The listing builds one solid part. Answer for the finished solid, in the listing's coordinates (mm). A direction names the side the tool comes from. Round coordinates to 2 decimals unless told otherwise and drop trailing zeros. Loops run counter-clockwise (first coordinate to the right, second up) from the corner with the lowest first, then second, coordinate; pieces in that order, holes last. Notation, with made-up numbers: (0.5, 37) -> (19.5, 37) arc R33 cw to (19.5, 69) -> close; hole circle Ø7 at (2.25, 82.25). An arc over 180 degrees is marked (long way). Use a Markdown table: item, result. Add a question column.
Q1. Which of the six approach directions +Z, -Z, +X, -X, +Y, -Y give full straight-line access (tool end or side, diameter ignored) to faces 5 (the flat face through (-5, 6.6, -4)), 6 (the flat face through (-4.5, 27, 4)), 7 (the cylindrical face through (-0.74, 9, 3.32))?
Q2. Section A-A on y = 36 is taken. Give the vertices of the cut face in (x, z).
Q3. Given pin 1 Ø1 at (x, y) = (-1.5, 31.5) entering from +Z; pin 2 Ø11 at (y, z) = (36, 0) entering from +X; pin 3 Ø10 at (y, z) = (16.5, 2.5) entering from +X; pin 4 Ø5 at (x, y) = (-2, 10) entering from -Z, each flat-ended and moving along its own axis, determine where each tip first touches the part or whether it passes through.
Q4. Section B-B on y = 3.5 is taken. Give the vertices of the cut face in (x, z) (3 decimals), then the cut area to 3 significant figures.
Q5. For a pull along Z with two mould halves and no side action, classify faces 1 (the flat face through (-5.193, 21.561, -0.061)), 2 (the flat face through (-4.25, 41, 6)), 3 (the cylindrical face through (0.1, 3, 7.9)), 4 (the cylindrical face through (-0.275, 15.016, -6.244)) as released by +Z, released by -Z, zero draft, split by the parting line, or undercut.
Q6. Section C-C on y = 14 is taken. Give the vertices of the cut face in (x, z).
Q7. Consider line 1 (Y direction, x = 3.75, z = -5.75); line 2 (X direction, y = 27, z = -4.25); line 3 (Y direction, x = 4.45, z = 0). Determine where each line is inside the solid, lowest interval first.
from build123d import *

# Parameters (mm, degrees)
SKETCH2_OUTSIDE_W        = 37.758
SKETCH2_OUTSIDE_H        = 37.758
CUT_EXTRUDE1_DEPTH       = 6.6
SKETCH3_OUTSIDE_W        = 37.758
SKETCH3_OUTSIDE_H        = 37.758
SKETCH3_OUTSIDE_W_2      = 9
SKETCH3_OUTSIDE_H_2      = 24
CUT_EXTRUDE2_DEPTH       = 31.630866785
SKETCH4_R                = 9.25
SKETCH4_R_2              = 7.25
CUT_EXTRUDE3_DEPTH       = 0.25
CUT_EXTRUDE4_START       = -0.25
SKETCH5_R                = 9.25
SKETCH5_R_2              = 7.25
CUT_EXTRUDE4_DEPTH       = 0.25
DOME2_FACE_RADIUS        = 7.25
DOME2_HEIGHT             = 3.8
FILLET1_R                = 1
FILLET2_R                = 0.25
CUT_EXTRUDE10_DEPTH      = 10.2995
M8_TAPPED_HOLE1_D        = 6.8
M8_TAPPED_HOLE1_DEPTH    = 22.25
M8_TAPPED_HOLE1_TIP      = 2.042926105
CUT_EXTRUDE11_DEPTH      = 51.168615687
CUT_EXTRUDE11_DEPTH_BACK = 51.168615687
SKETCH6_R                = 7.25


# Read off the part's stored shape, not the designer's step: Dome1
with BuildPart() as part:
    # Sketch1 → Revolve1 (revolve)
    with BuildSketch(Plane(origin=(0, 0, 0), x_dir=(0, 0, -1), z_dir=(1, 0, 0)), mode=Mode.PRIVATE) as revolve1_sk:
        with BuildLine():
            Line((0, 0), (7.9, 0))
            Line((7.9, 0), (7.9, 6.6))
            Line((7.9, 6.6), (6.25, 6.6))
            Line((6.25, 6.6), (6.25, 23.2))
            Line((6.25, 23.2), (10.245555029, 29.752712416))
            ThreePointArc((10.245555029, 29.752712416), (10.463447114, 41.875055276), (0, 48))
            Line((0, 48), (0, 0))
        make_face()
    revolve(revolve1_sk.sketch.rotate(Axis((0, 48, 0), (0, -1, 0)), 180), axis=Axis((0, 48, 0), (0, -1, 0)))

    # Sketch2 outside → Cut-Extrude1 (cut)
    with BuildSketch(Plane(origin=(0, 0, 0), x_dir=(-1, 0, 0), z_dir=(0, -1, 0))):
        Rectangle(SKETCH2_OUTSIDE_W, SKETCH2_OUTSIDE_H)
        with BuildLine():
            Line((-6.925, 3.801890977), (-6.925, -3.801890977))
            ThreePointArc((-6.925, -3.801890977), (0, -7.9), (6.925, -3.801890977))
            Line((6.925, -3.801890977), (6.925, 3.801890977))
            ThreePointArc((6.925, 3.801890977), (0, 7.9), (-6.925, 3.801890977))
        make_face(mode=Mode.SUBTRACT)
    extrude(amount=-CUT_EXTRUDE1_DEPTH, mode=Mode.SUBTRACT)

    # Sketch3 outside → Cut-Extrude2 (cut, through all)
    with BuildSketch(Plane(origin=(0, 22.5, 0), x_dir=(-1, 0, 0), z_dir=(0, -1, 0))):
        Rectangle(SKETCH3_OUTSIDE_W, SKETCH3_OUTSIDE_H)
        Rectangle(SKETCH3_OUTSIDE_W_2, SKETCH3_OUTSIDE_H_2, mode=Mode.SUBTRACT)
    extrude(amount=-CUT_EXTRUDE2_DEPTH, mode=Mode.SUBTRACT)

    # Sketch4 → Cut-Extrude3 (cut)
    with BuildSketch(Plane(origin=(4.5, 0, 0), x_dir=(0, 0, -1), z_dir=(1, 0, 0))):
        with Locations((0, 36)):
            Circle(SKETCH4_R)
        with Locations((0, 36)):
            Circle(SKETCH4_R_2, mode=Mode.SUBTRACT)
    extrude(amount=-CUT_EXTRUDE3_DEPTH, mode=Mode.SUBTRACT)

    # Sketch5 → Cut-Extrude4 (cut)
    with BuildSketch(Plane.ZY.offset(4.5).offset(CUT_EXTRUDE4_START)):
        with Locations(Location((0, 36, 0), (0, 0, 180))):
            Circle(SKETCH5_R)
        with Locations(Location((0, 36, 0), (0, 0, 180))):
            Circle(SKETCH5_R_2, mode=Mode.SUBTRACT)
    extrude(amount=CUT_EXTRUDE4_DEPTH, mode=Mode.SUBTRACT)

    # Dome1 outline → Dome1 (revolve)
    with BuildSketch(Plane(origin=(0, 36, 0), x_dir=(0, 1, 0), z_dir=(0, 0, -1))):
        with BuildLine():
            Line((0, -4.499999993), (0, -8.3))
            ThreePointArc((0, -8.3), (4.092752745, -7.292422991), (7.250000005, -4.499999993))
            Line((7.250000005, -4.499999993), (0, -4.499999993))
        make_face()
    revolve(axis=Axis((0, 36, 0), (1, 0, 0)))

    # Dome2: a dome of height H over a round flat face of radius A is a cap of a sphere of radius (A * A + H * H) / (2 * H)
    dome2_r = (DOME2_FACE_RADIUS * DOME2_FACE_RADIUS + DOME2_HEIGHT * DOME2_HEIGHT) / (2 * DOME2_HEIGHT)
    dome2_base = Plane((4.5, 36, 0), z_dir=(1, 0, 0))
    with Locations(dome2_base.offset(DOME2_HEIGHT - dome2_r)):
        dome2_ball = Sphere(dome2_r, mode=Mode.PRIVATE)
    add(split(dome2_ball, bisect_by=dome2_base, keep=Keep.TOP, mode=Mode.PRIVATE))

    # Fillet1
    # the kernel refuses this fillet: 1 mm, written as the material it takes off along each edge
    with BuildSketch(Plane(origin=(0, 6.6, 0), x_dir=(-0.9669082627273712, 0, 0.25512430591681584), z_dir=(0.25512430591681584, 0, 0.9669082627273712))) as fillet1_piece_1:
        with BuildLine():
            CenterArc((7.9 - FILLET1_R, FILLET1_R), FILLET1_R, 270, 90)
            Line((7.9, FILLET1_R), (7.9 + FILLET1_R * 0.02, FILLET1_R))
            Line((7.9 + FILLET1_R * 0.02, FILLET1_R), (7.9 + FILLET1_R * 0.02, -FILLET1_R * 0.02))
            Line((7.9 + FILLET1_R * 0.02, -FILLET1_R * 0.02), (7.9 - FILLET1_R, -FILLET1_R * 0.02))
            Line((7.9 - FILLET1_R, -FILLET1_R * 0.02), (7.9 - FILLET1_R, 0))
        make_face()
    revolve(axis=Axis((0, 6.6, 0), (0, -1, 0)), revolution_arc=209.561901965, mode=Mode.SUBTRACT)
    with BuildSketch(Plane(origin=(0, 6.6, 0), x_dir=(-0.9669082627273712, 0, -0.2551243059168157), z_dir=(0.2551243059168157, 0, -0.9669082627273712))) as fillet1_piece_2:
        with BuildLine():
            CenterArc((7.9 - FILLET1_R, -FILLET1_R), FILLET1_R, 360, 90)
            Line((7.9, -FILLET1_R), (7.9 + FILLET1_R * 0.02, -FILLET1_R))
            Line((7.9 + FILLET1_R * 0.02, -FILLET1_R), (7.9 + FILLET1_R * 0.02, FILLET1_R * 0.02))
            Line((7.9 + FILLET1_R * 0.02, FILLET1_R * 0.02), (7.9 - FILLET1_R, FILLET1_R * 0.02))
            Line((7.9 - FILLET1_R, FILLET1_R * 0.02), (7.9 - FILLET1_R, 0))
        make_face()
    revolve(axis=Axis((0, 6.6, 0), (0, 1, 0)), revolution_arc=209.561901965, mode=Mode.SUBTRACT)

    # Fillet2
    fillet2_edges = [part.edges().sort_by_distance(p)[0] for p in [
        (0, 0, -7.9),
        (0, 0, 7.9),
        (6.925, 0, 0),
        (-6.925, 0, 0),
    ]]
    fillet(fillet2_edges, radius=FILLET2_R)

    # Sketch11 → Cut-Extrude10 (cut, symmetric)
    with BuildSketch(Plane(origin=(0, 0, 0), x_dir=(-1, 0, 0), z_dir=(0, 0, -1))):
        Polygon((-6.25, 22.5), (-4.5, 22.5), (-6.25, 20.127174391), align=None)
        Polygon((4.5, 22.5), (6.25, 22.5), (6.25, 20.127174391), align=None)
    extrude(amount=CUT_EXTRUDE10_DEPTH, both=True, mode=Mode.SUBTRACT)

    # M8 Tapped Hole1
    with Locations(Plane(origin=(0, -4.5, 0), x_dir=(-1, 0, 0), z_dir=(0, -1, 0))):
        with Locations((0, 0)):
            Hole(M8_TAPPED_HOLE1_D / 2, depth=M8_TAPPED_HOLE1_DEPTH)
            with Locations((0, 0, -(M8_TAPPED_HOLE1_DEPTH + M8_TAPPED_HOLE1_TIP / 2))):  # 118° drill point
                Cone(0, M8_TAPPED_HOLE1_D / 2, M8_TAPPED_HOLE1_TIP, mode=Mode.SUBTRACT)

    # Sketch6 → Cut-Extrude11 (cut, two sides: drawn at the far end of the back side and taken through both)
    with BuildSketch(Plane(origin=(0, 0, 0), x_dir=(0, 0, -1), z_dir=(1, 0, 0)).offset(-CUT_EXTRUDE11_DEPTH_BACK)):
        with Locations((0, 36)):
            Circle(SKETCH6_R)
    extrude(amount=CUT_EXTRUDE11_DEPTH + CUT_EXTRUDE11_DEPTH_BACK, mode=Mode.SUBTRACT)


solid = part.part
Checked values:
| question | item | result |
|---|---|---|
| 1 | face 5 | none |
| 1 | face 6 | +Z, -Z, -X, +Y |
| 1 | face 7 | -Y |
| 2 | outline | (-4.5, -11.12) arc R12 ccw to (4.5, -11.12) -> (4.5, -9.25) -> (4.25, -9.25) -> (4.25, -7.25) -> (-4.25, -7.25) -> (-4.25, -9.25) -> (-4.5, -9.25) -> close; (-4.5, 9.25) -> (-4.25, 9.25) -> (-4.25, 7.25) -> (4.25, 7.25) -> (4.25, 9.25) -> (4.5, 9.25) -> (4.5, 11.12) arc R12 ccw to (-4.5, 11.12) -> close |
| 3 | pin 1 | stops at z = 11.22 |
| 3 | pin 2 | passes through |
| 3 | pin 3 | stops at x = 6.25 |
| 3 | pin 4 | stops at z = -6.25 |
| 4 | outline | (-6.925, -3.802) arc R7.9 ccw to (6.925, -3.802) -> (6.925, 3.802) arc R7.9 ccw to (-6.925, 3.802) -> close; hole circle Ø6.8 at (0, 0) |
| 4 | area | 150 mm2 |
| 5 | face 1 | zero draft |
| 5 | face 2 | undercut |
| 5 | face 3 | released by +Z |
| 5 | face 4 | split by the parting line |
| 6 | outline | circle Ø12.5 at (0, 0); hole circle Ø6.8 at (0, 0) |
| 7 | line 1 | y = 0 to 6.6, 24.21 to 31.58, 40.42 to 45.84 |
| 7 | line 2 | x = -4.5 to 4.5 |
| 7 | line 3 | y = 0 to 26.75, 45.25 to 47.14 |
